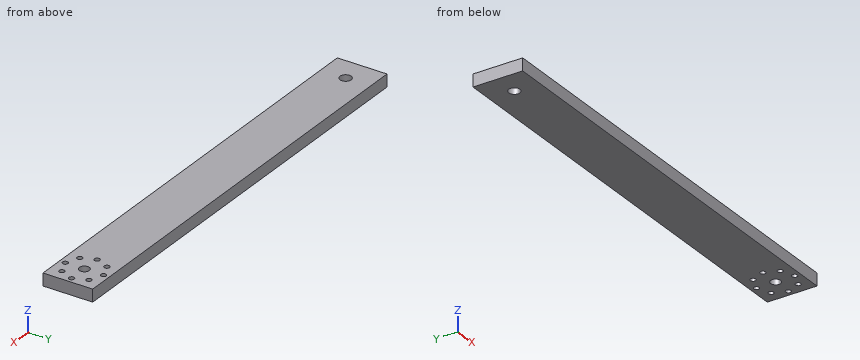
Autodesk Inventor part; units mm, degrees
ref_plane "YZ Plane" through (0, 0, 0) normal (1, 0, 0) x (0, 1, 0)
ref_plane "XZ Plane" through (0, 0, 0) normal (0, 1, 0) x (-1, 0, 0)
ref_plane "XY Plane" through (0, 0, 0) normal (0, 0, 1) x (1, 0, 0)
sketch "Sketch1" plane through (0, 0, 0) normal (0, 0, 1) x (1, 0, 0)
  line L0 (0, 0) -> (225.806, 0)
  line L1 (225.806, 0) -> (225.806, 25.4)
  line L2 (225.806, 25.4) -> (0, 25.4)
  line L3 (0, 25.4) -> (0, 0)
  dimension "d0" = 225.806
  dimension "d1" = 25.4
extrude "Extrusion1" add sketch "Sketch1" along normal blind 6.35
sketch "Sketch2" plane through (0, 0, 6.35) normal (0, 0, 1) x (1, 0, 0)
  line L0 (0, 25.4) -> (0, 0)
  line L1 (0, 0) -> (225.806, 0)
  line L2 (225.806, 25.4) -> (0, 25.4)
  circle A0 centre (12.7, 12.7) radius 2.8829
  dimension "d4" = 12.7
  dimension "d5" = 25.4
  dimension "d6" = 5.7658
  dimension "d15" = 12.7
extrude "Extrusion2" cut sketch "Sketch2" against normal through all
sketch "Sketch3" plane through (0, 0, 6.35) normal (0, 0, 1) x (1, 0, 0)
  line L0 (0, 0) -> (225.806, 0)
  line L1 (225.806, 25.4) -> (0, 25.4)
  line L2 (225.806, 0) -> (225.806, 25.4)
  circle A0 centre (213.106, 12.7) radius 2.54
  dimension "d9" = 25.4
  dimension "d10" = 12.7
  dimension "d11" = 12.7
  dimension "d12" = 5.08
extrude "Extrusion3" cut sketch "Sketch3" against normal through all
sketch "Sketch4" plane through (0, 0, 6.35) normal (0, 0, 1) x (1, 0, 0)
  circle A0 centre (213.106, 12.7) radius 2.54
  circle A1 centre (213.106, 12.7) radius 9.779
  line L0 (213.106, 22.479) -> (206.1847, 19.6083)
  line L1 (206.1847, 19.6083) -> (203.327, 12.7)
  line L2 (203.327, 12.7) -> (206.1977, 5.7787)
  line L3 (206.1977, 5.7787) -> (213.106, 2.921)
  line L4 (213.106, 2.921) -> (220.0273, 5.7917)
  line L5 (220.0273, 5.7917) -> (222.885, 12.7)
  line L6 (222.885, 12.7) -> (220.0143, 19.6213)
  line L7 (220.0143, 19.6213) -> (213.106, 22.479)
  circle A2 centre (213.106, 22.479) radius 1.3589
  circle A3 centre (220.0143, 19.6213) radius 1.3589
  circle A4 centre (222.885, 12.7) radius 1.3589
  circle A5 centre (220.0273, 5.7917) radius 1.3589
  circle A6 centre (213.106, 2.921) radius 1.3589
  circle A7 centre (206.1977, 5.7787) radius 1.3589
  circle A8 centre (203.327, 12.7) radius 1.3589
  circle A9 centre (206.1847, 19.6083) radius 1.3589
  point P0 (0, 0)
  dimension "d16" = 19.558
  dimension "d17" = 7.493
  dimension "d18" = 2.7178
  dimension "d19" = 2.7178
  dimension "d20" = 2.7178
  dimension "d21" = 2.7178
  dimension "d22" = 2.7178
  dimension "d23" = 2.7178
  dimension "d24" = 2.7178
  dimension "d25" = 2.7178
extrude "Extrusion4" cut sketch "Sketch4" against normal through all contours L6 A4 A1 | A1 A4 | A1 A4 L5 | L5 A4 L6 | A3 L6 A1 | A1 A3 | A5 A1 | A1 L5 A5 | L5 L4 A5 | A3 L7 L6 | L7 A3 A1 | A1 A5 L4 | A6 A1 L4 | L4 L3 A6 | A2 L0 L7 | L7 A1 A2 | A1 A2 | A6 A1 | A1 A6 L3 | L0 A2 A1 | A7 A1 L3 | L3 L2 A7 | A9 L1 L0 | L0 A1 A9 | A7 A1 | A1 A7 L2 | A1 A9 | L1 A9 A1 | A8 A1 | A1 L2 A8 | L2 L1 A8 | A8 L1 A1
equation "\"d15\" = 0.5 * d5"
equation "\"d19\" = d18"
equation "\"d20\" = d18"
equation "\"d21\" = d18"
equation "\"d22\" = d18"
equation "\"d23\" = d18"
equation "\"d24\" = d18"
equation "\"d25\" = d18"
properties part number "bar arms"
CAD build for the part. Positions are in the model's coordinates, mm. Round coordinates to 2 decimals unless told otherwise and drop trailing zeros. Write each loop counter-clockwise with the first axis right and the second up, starting at its lowest first coordinate (ties: lowest second). Pieces come first, ordered by that corner, then holes.
(1) Slice it at A-A, the plane x = 12.7. Write the cut outline in (y, z).
(2) Drop flat-ended pins along their axis: P1, Ø6, axis at x = 30.5, y = 7, coming from the -Z side; P2, Ø2.5, axis at x = 213.106, y = 22.479, coming from the +Z side. Give the stop position or say it passes through.
(3) Probe line 1 along Y through (x, z) = (212.5, 1.5); line 2 along X through (y, z) = (13.25, 3.75); line 3 along X through (y, z) = (2.75, 4.75). List the from-to ranges inside material, lowest first.
(4) Slice it at B-B, the plane z = 4. Count the separate pieces of the cut face and the enclosed holes in it, and give its area (3 significant figures).
From the geometry:
1. outline: (0, 0) - (9.82, 0) - (9.82, 6.35) - (0, 6.35) - close; (15.58, 0) - (25.4, 0) - (25.4, 6.35) - (15.58, 6.35) - close
2. P1: stops at z = 0
2. P2: passes through
3. line 1: y = 0 to 1.7, 4.14 to 10.23, 15.17 to 21.26, 23.7 to 25.4
3. line 2: x = 0 to 9.87, 15.53 to 202.08, 204.57 to 210.63, 215.59 to 221.64, 224.13 to 225.81
3. line 3: x = 0 to 211.76, 214.45 to 225.81
4. separate pieces: 1
4. enclosed holes: 10
4. area: 5,640 mm2
